Can you work these out from the model? Positions are in its coordinate system, mm. Give positions to 0.01 mm unless a question says otherwise; leave off trailing zeros. Order: outer loops, then holes, each group sorted by start corner. A loop starts at its lowest first (then second) coordinate and runs counter-clockwise, first axis right, second up. Notation, with made-up numbers: (52.25, 47) - (91.25, 47) arc R15 ccw to (91.25, 56) - close; hole circle Ø8 at (30, -3). An arc over 180 degrees is marked (long way). Return JSON: item names as keys, results as strings.
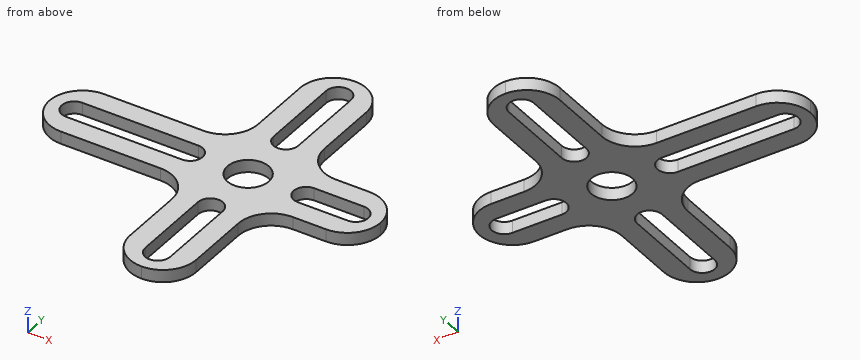
```python
from build123d import *

# Parameters (mm, degrees)
EXTRUDE_2_DEPTH     = 1.5
FILLET_1_DEPTH      = 1.5
FILLET_1_2_DEPTH    = 1.5
SKETCH_3_R          = 2.5
CUT_EXTRUDE_2_DEPTH = 1.5
FILLET_2_R          = 4


with BuildPart() as part:
    # 草图1 → 凸台-拉伸2 (new body)
    with BuildSketch(Plane.XY):
        Polygon((-24, 4), (-4, 4), (-4, 19.75), (4, 19.75), (4, 4), (16, 4), (16, -4), (4, -4), (4, -19.75), (-4, -19.75), (-4, -4), (-24, -4), align=None)
        with BuildLine():
            Line((-21, 1.5), (-7, 1.5))
            ThreePointArc((-7, 1.5), (-5.5, 0), (-7, -1.5))
            Line((-7, -1.5), (-21, -1.5))
            ThreePointArc((-21, -1.5), (-22.5, 0), (-21, 1.5))
        make_face(mode=Mode.SUBTRACT)
        with BuildLine():
            Line((7, 1.5), (13, 1.5))
            ThreePointArc((13, 1.5), (14.5, 0), (13, -1.5))
            Line((13, -1.5), (7, -1.5))
            ThreePointArc((7, -1.5), (5.5, 0), (7, 1.5))
        make_face(mode=Mode.SUBTRACT)
        with BuildLine():
            Line((-1.5, -16.75), (-1.5, -7))
            ThreePointArc((-1.5, -7), (0, -5.5), (1.5, -7))
            Line((1.5, -7), (1.5, -16.75))
            ThreePointArc((1.5, -16.75), (0, -18.25), (-1.5, -16.75))
        make_face(mode=Mode.SUBTRACT)
        with BuildLine():
            Line((1.5, 16.75), (1.5, 7))
            ThreePointArc((1.5, 7), (0, 5.5), (-1.5, 7))
            Line((-1.5, 7), (-1.5, 16.75))
            ThreePointArc((-1.5, 16.75), (0, 18.25), (1.5, 16.75))
        make_face(mode=Mode.SUBTRACT)
    extrude(amount=EXTRUDE_2_DEPTH)

    # 圆角1: read off the stored shape, not the designer's step
    # 圆角1 outline → 圆角1 (cut)
    with BuildSketch(Plane.XY):
        with BuildLine():
            ThreePointArc((4, -15.75), (2.828427125, -18.578427125), (0, -19.75))
            Line((0, -19.75), (4, -19.75))
            Line((4, -19.75), (4, -15.75))
        make_face()
        with BuildLine():
            ThreePointArc((0, -19.75), (-2.828427125, -18.578427125), (-4, -15.75))
            Line((-4, -15.75), (-4, -19.75))
            Line((-4, -19.75), (0, -19.75))
        make_face()
        with BuildLine():
            ThreePointArc((-4, 15.75), (-2.828427125, 18.578427125), (0, 19.75))
            Line((0, 19.75), (-4, 19.75))
            Line((-4, 19.75), (-4, 15.75))
        make_face()
        with BuildLine():
            ThreePointArc((0, 19.75), (2.828427125, 18.578427125), (4, 15.75))
            Line((4, 15.75), (4, 19.75))
            Line((4, 19.75), (0, 19.75))
        make_face()
    extrude(amount=FILLET_1_DEPTH, mode=Mode.SUBTRACT)

    # Fillet 1 2 outline → Fillet 1 2 (add)
    with BuildSketch(Plane.XY):
        with BuildLine():
            Line((4, -4), (4, -8))
            ThreePointArc((4, -8), (5.171572875, -5.171572875), (8, -4))
            Line((8, -4), (4, -4))
        make_face()
        with BuildLine():
            ThreePointArc((-8, -4), (-5.171572875, -5.171572875), (-4, -8))
            Line((-4, -8), (-4, -4))
            Line((-4, -4), (-8, -4))
        make_face()
        with BuildLine():
            Line((-4, 4), (-4, 8))
            ThreePointArc((-4, 8), (-5.171572875, 5.171572875), (-8, 4))
            Line((-8, 4), (-4, 4))
        make_face()
        with BuildLine():
            ThreePointArc((8, 4), (5.171572875, 5.171572875), (4, 8))
            Line((4, 8), (4, 4))
            Line((4, 4), (8, 4))
        make_face()
    extrude(amount=FILLET_1_2_DEPTH)

    # 草图3 → 切除-拉伸2 (cut)
    with BuildSketch(Plane.XY.offset(1.5)):
        Circle(SKETCH_3_R)
    extrude(amount=-CUT_EXTRUDE_2_DEPTH, mode=Mode.SUBTRACT)

    # 圆角2
    fillet_2_edges = [part.edges().sort_by_distance(p)[0] for p in [
        (-24, -4, 0.75),
        (-24, 4, 0.75),
        (16, -4, 0.75),
        (16, 4, 0.75),
    ]]
    fillet(fillet_2_edges, radius=FILLET_2_R - 0.0001)  # a hair under: the kernel refuses the full size


solid = part.part
```
1. Suppose I cut it at C-C (z = 0.75). State how many separate pieces and enclosed holes the cut face has, plus the area to 3 significant figures.
Checks:
{"separate pieces": "1", "enclosed holes": "5", "area": "392 mm^2"}
2. Suppose I cut it at D-D (y = -3). List the corners of the cut face in (x, z) for me.
Checks:
{"outline": "(-22.65, 0) - (14.65, 0) - (14.65, 1.5) - (-22.65, 1.5) - close"}
3. For pin 1 Ø3 at (x, y) = (-6.5, -8) entering from +Z, with a flat end and sliding along its axis, tell me the tip position at first contact or that it passes through.
Checks:
{"pin 1": "through"}
4. If I drill on L1, parallel to X at y = 15.5, z = 0.15; L2, parallel to X at y = 18.5, z = 0.6, over which ranges is the centre line in solid material (lowest first)? Write a range as [from, to].
Checks:
{"L1": "[-4, -1.5], [1.5, 4]", "L2": "[-2.9, 2.9]"}
5. Suppose I cut it at A-A (y = 13.5). List the corners of the cut face in (x, z) for me.
Checks:
{"outline": "(-4, 0) - (-1.5, 0) - (-1.5, 1.5) - (-4, 1.5) - close; (1.5, 0) - (4, 0) - (4, 1.5) - (1.5, 1.5) - close"}
